from build123d import *

# Parameters (mm, degrees)
F0_W           = 50
F0_H           = 65
F1_DEPTH       = 6
F2_W           = 15
F2_H           = 10
F3_DEPTH       = 41
F5_D           = 3.2
F5_CBORE_D     = 6
F5_CBORE_DEPTH = 3.5
F7_D           = 2.2


with BuildPart() as f1:
    # F0 (on Top) → F1 (new body)
    with BuildSketch(Plane.XY):
        with Locations((25, 32.5)):
            Rectangle(F0_W, F0_H)
    extrude(amount=F1_DEPTH)

    # F2 (on face) → F3 (join)
    with BuildSketch(Plane.XY.offset(6)):
        with Locations((25, 55)):
            Rectangle(F2_W, F2_H)
    extrude(amount=F3_DEPTH)

    # F5 (through all)
    with Locations(Plane.XY.offset(6)):
        with Locations((12, 55), (38, 55), (25, 32.48334)):
            CounterBoreHole(F5_D / 2, F5_CBORE_D / 2, F5_CBORE_DEPTH)

    # F7 (through all)
    with Locations(Plane.XY.offset(6)):
        with Locations((11, 25), (39, 25), (39, 5), (11, 5), (44.5, 35)):
            Hole(F7_D / 2)


solid = f1.part
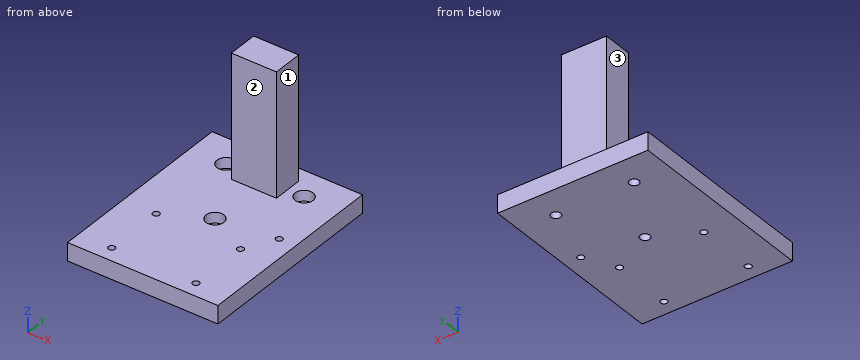
Geometry: final body of the model. Coordinates: model frame, mm. Face numbers are marked on the shaded views. A direction names the side the tool comes from. Round coordinates to 2 decimals unless told otherwise and drop trailing zeros. Loops run counter-clockwise (first coordinate to the right, second up) from the corner with the lowest first, then second, coordinate; pieces in that order, holes last.
Q1. Section D-D on x = 44.5. Return loops of the section in (y, z), plus the area to 3 significant figures.
Q2. Pin query (flat end, axial travel): P1, Ø4.5, axis at x = 26, z = 28.5, coming from the +Y side; P2, Ø12, axis at x = 7.5, y = 23, coming from the +Z side; P3, Ø1.9, axis at x = 12, y = 55, coming from the -Z side; P4, Ø4, axis at x = 25, y = 32.48, coming from the +Z side. Return the tip coordinate at first contact, or that it passes through.
Q3. Access query for the marked faces 1, 2 and 3. Directions: +Z, -Z, +X, -X, +Y, -Y. A direction counts if a zero-diameter tool reaches every point of the face in a straight line with its end or side. Return the directions, or none.
Q4. Section A-A on x = 25. Return loops of the section in (y, z).
Q5. Section B-B on y = 55. Return loops of the section in (x, z), plus the area to 3 significant figures.
Q6. Section C-C on y = 25. Return loops of the section in (x, z), plus the area to 3 significant figures.
Q7. Material intervals for L1, parallel to Y at x = 25, z = 4.5; L2, parallel to Y at x = 44.5, z = 2.25; L3, parallel to Y at x = 39, z = 4, sorted ascending.
Evaluation:
1. outline: (0, 0) - (33.9, 0) - (33.9, 6) - (0, 6) - close; (36.1, 0) - (65, 0) - (65, 6) - (36.1, 6) - close
1. area: 377 mm2
2. P1: stops at y = 60
2. P2: stops at z = 6
2. P3: passes through
2. P4: stops at z = 2.5
3. face 1: +Z, +X, +Y, -Y
3. face 2: +Z, +X, -X, -Y
3. face 3: +Z, -X, +Y, -Y
4. outline: (0, 0) - (30.88, 0) - (30.88, 2.5) - (29.48, 2.5) - (29.48, 6) - (0, 6) - close; (34.08, 0) - (65, 0) - (65, 6) - (60, 6) - (60, 47) - (50, 47) - (50, 6) - (35.48, 6) - (35.48, 2.5) - (34.08, 2.5) - close
5. outline: (0, 0) - (10.4, 0) - (10.4, 2.5) - (9, 2.5) - (9, 6) - (0, 6) - close; (13.6, 0) - (36.4, 0) - (36.4, 2.5) - (35, 2.5) - (35, 6) - (32.5, 6) - (32.5, 47) - (17.5, 47) - (17.5, 6) - (15, 6) - (15, 2.5) - (13.6, 2.5) - close; (39.6, 0) - (50, 0) - (50, 6) - (41, 6) - (41, 2.5) - (39.6, 2.5) - close
5. area: 857 mm2
6. outline: (0, 0) - (9.9, 0) - (9.9, 6) - (0, 6) - close; (12.1, 0) - (37.9, 0) - (37.9, 6) - (12.1, 6) - close; (40.1, 0) - (50, 0) - (50, 6) - (40.1, 6) - close
6. area: 274 mm2
7. L1: y = 0 to 29.48, 35.48 to 65
7. L2: y = 0 to 33.9, 36.1 to 65
7. L3: y = 0 to 3.9, 6.1 to 23.9, 26.1 to 52.17, 57.83 to 65
